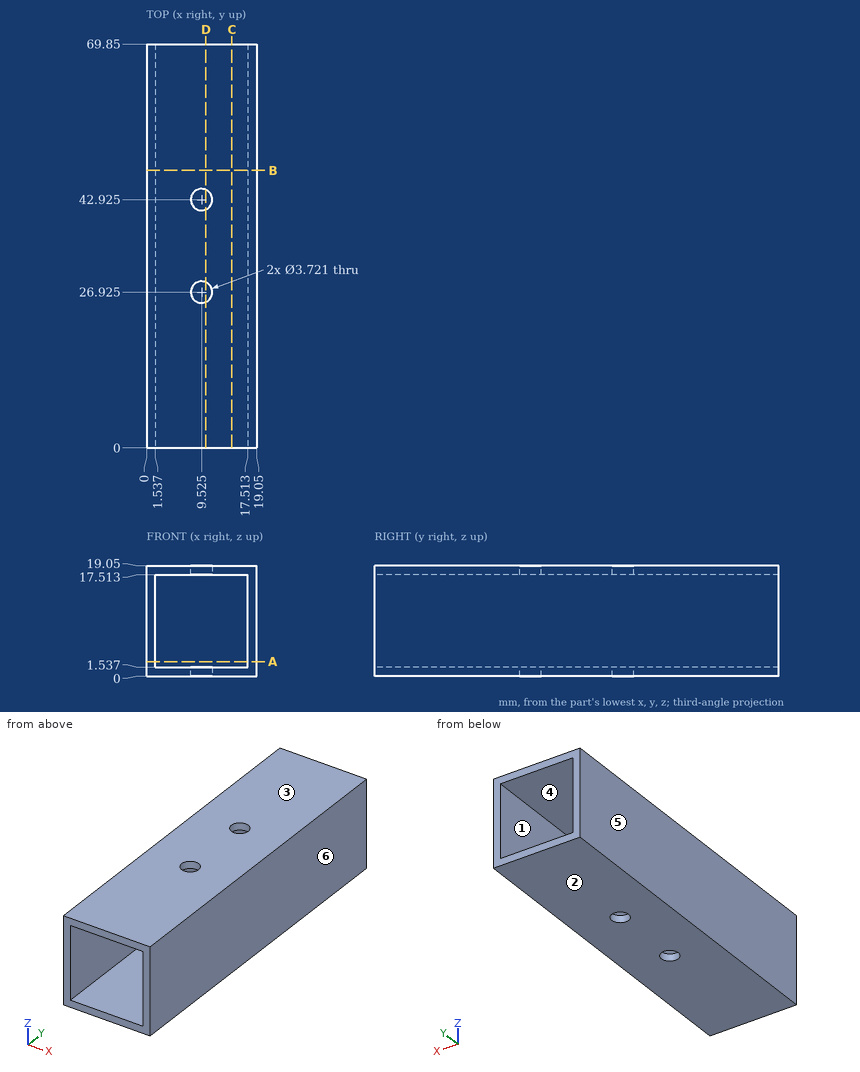
Source: three-view drawing plus pictorial views. Frame: mm from the lowest corner of the part. A direction names the side the tool comes from. Coordinates: 2 decimals unless noted, no trailing zeros. Order: outer loops, then holes, each group sorted by start corner. A loop starts at its lowest first (then second) coordinate and runs counter-clockwise, first axis right, second up. Notation, with made-up numbers: (36, 13.5) -> (63, 13.5) arc R18 ccw to (63, 31.5) -> close; hole circle Ø6 at (63.25, 75). An arc over 180 degrees is marked (long way). Write item = value, one per line.
(1) Cut plane D-D on x = 10.25. Return loops of the section in (y, z).
Solved:
outline = (0, 0) -> (25.21, 0) -> (25.21, 1.54) -> (0, 1.54) -> close; (0, 17.51) -> (25.21, 17.51) -> (25.21, 19.05) -> (0, 19.05) -> close; (28.64, 0) -> (41.21, 0) -> (41.21, 1.54) -> (28.64, 1.54) -> close; (28.64, 17.51) -> (41.21, 17.51) -> (41.21, 19.05) -> (28.64, 19.05) -> close; (44.64, 0) -> (69.85, 0) -> (69.85, 1.54) -> (44.64, 1.54) -> close; (44.64, 17.51) -> (69.85, 17.51) -> (69.85, 19.05) -> (44.64, 19.05) -> close
(2) Pull-direction query (X, two-part tool) for the marked faces 3, 4, 5 and 6; classes: pulls with the +X half, pulls with the -X half, needs draft (parallel to the pull), parting line crosses it, or undercut.
Solved:
face_3 = needs draft
face_4 = undercut
face_5 = pulls with the -X half
face_6 = pulls with the +X half
(3) Pin query (flat end, axial travel): pin 1 Ø2 at (x, z) = (15.5, 16) entering from +Y. Return the tip coordinate at first contact, or that it passes through.
Solved:
pin_1 = through
(4) Cut plane C-C on x = 14.75. Return loops of the section in (y, z).
Solved:
outline = (0, 0) -> (69.85, 0) -> (69.85, 1.54) -> (0, 1.54) -> close; (0, 17.51) -> (69.85, 17.51) -> (69.85, 19.05) -> (0, 19.05) -> close
(5) Access query for the marked faces 1 and 2. Directions: +Z, -Z, +X, -X, +Y, -Y. A direction counts if a zero-diameter tool reaches every point of the face in a straight line with its end or side. Return the directions, or none.
Solved:
face_1 = +Y, -Y
face_2 = -Z, +X, -X, +Y, -Y
(6) Cut plane A-A on z = 2.5. Return loops of the section in (x, y), plus the area to 3 significant figures.
Solved:
outline = (0, 0) -> (1.54, 0) -> (1.54, 69.85) -> (0, 69.85) -> close; (17.51, 0) -> (19.05, 0) -> (19.05, 69.85) -> (17.51, 69.85) -> close
area = 215 mm²
(7) Cut plane B-B on y = 48. Return loops of the section in (x, z), plus the area to 3 significant figures.
Solved:
outline = (0, 0) -> (19.05, 0) -> (19.05, 19.05) -> (0, 19.05) -> close; hole (1.54, 1.54) -> (17.51, 1.54) -> (17.51, 17.51) -> (1.54, 17.51) -> close
area = 108 mm²
(8) Line query: line 1 (X direction, y = 34.5, z = 3). Output: solid intervals per line, ascending.
Solved:
line_1 = 0 to 1.54, 17.51 to 19.05
